from build123d import *

# Parameters (mm, degrees)
SKETCH1_R           = 15
BOSS_EXTRUDE1_DEPTH = 15


with BuildPart() as part:
    # Sketch1 → Boss-Extrude1 (new, symmetric)
    with BuildSketch(Plane.XY):
        with BuildLine():
            Line((0, 0), (0, 106))
            ThreePointArc((0, 106), (1.171572875, 108.828427125), (4, 110))
            Line((4, 110), (56, 110))
            ThreePointArc((56, 110), (58.828427125, 108.828427125), (60, 106))
            Line((60, 106), (60, 83.851648071))
            ThreePointArc((60, 83.851648071), (61.068687565, 81.129992802), (63.703703704, 79.862637103))
            ThreePointArc((63.703703704, 79.862637103), (95.355339059, 65.355339059), (109.862637103, 33.703703704))
            ThreePointArc((109.862637103, 33.703703704), (111.129992802, 31.068687565), (113.851648071, 30))
            Line((113.851648071, 30), (151, 30))
            ThreePointArc((151, 30), (153.828427125, 28.828427125), (155, 26))
            Line((155, 26), (155, 0))
            Line((155, 0), (0, 0))
        make_face()
        with Locations((30, 80)):
            Circle(SKETCH1_R, mode=Mode.SUBTRACT)
        with BuildLine():
            Line((85.690465157, 30), (24, 30))
            ThreePointArc((24, 30), (21.171572875, 31.171572875), (20, 34))
            Line((20, 34), (20, 56))
            ThreePointArc((20, 56), (21.171572875, 58.828427125), (24, 60))
            Line((24, 60), (60, 60))
            ThreePointArc((60, 60), (79.513309068, 52.786635759), (89.642844412, 34.615384615))
            ThreePointArc((89.642844412, 34.615384615), (88.728683259, 31.398225458), (85.690465157, 30))
        make_face(mode=Mode.SUBTRACT)
    extrude(amount=BOSS_EXTRUDE1_DEPTH, both=True)


solid = part.part
Check sheet for the modelled part. Datum: model origin and axes. Units: mm. A direction names the side the tool comes from. Coordinates: 2 decimals unless noted, no trailing zeros. Loops run counter-clockwise (first coordinate to the right, second up) from the corner with the lowest first, then second, coordinate; pieces in that order, holes last. Notation, with made-up numbers: (34, 55.5) -> (60, 55.5) arc R25 ccw to (60, 81.5) -> close; hole circle Ø7 at (83.25, 75.25). An arc over 180 degrees is marked (long way). Answer in a Markdown table with one row per item.
1. Sectioned sample at D-D, the plane x = 132. Record the boundary of the cut face in (y, z), then the cut area to 3 significant figures.
Check values:
| item | result |
|---|---|
| outline | (0, -15) -> (30, -15) -> (30, 15) -> (0, 15) -> close |
| area | 900 mm2 |
2. Sectioned sample at C-C, the plane y = 47.5. Record the boundary of the cut face in (x, z), then the cut area to 3 significant figures.
Check values:
| item | result |
|---|---|
| outline | (0, -15) -> (20, -15) -> (20, 15) -> (0, 15) -> close; (84.37, -15) -> (106.84, -15) -> (106.84, 15) -> (84.37, 15) -> close |
| area | 1,270 mm2 |
3. Sectioned sample at B-B, the plane z = -6. Record the boundary of the cut face in (x, y), then the cut area to 3 significant figures.
Check values:
| item | result |
|---|---|
| outline | (0, 0) -> (155, 0) -> (155, 26) arc R4 ccw to (151, 30) -> (113.85, 30) arc R4 cw to (109.86, 33.7) arc R50 ccw to (63.7, 79.86) arc R4 cw to (60, 83.85) -> (60, 106) arc R4 ccw to (56, 110) -> (4, 110) arc R4 ccw to (0, 106) -> close; hole circle Ø30 at (30, 80); hole (20, 34) arc R4 ccw to (24, 30) -> (85.69, 30) arc R4 ccw to (89.64, 34.62) arc R30 ccw to (60, 60) -> (24, 60) arc R4 ccw to (20, 56) -> close |
| area | 8,810 mm2 |
4. Material ranges on line 1 along Y through (x, z) = (30, 3.75); line 2 along X through (y, z) = (73, 7); line 3 along X through (y, z) = (100.5, -6.75), recorded low to high. Write a range as [from, to].
Check values:
| item | result |
|---|---|
| line 1 | y = [0, 30], [60, 65], [95, 110] |
| line 2 | x = [0, 16.73], [43.27, 85.51] |
| line 3 | x = [0, 60] |
5. Access from +Z, -Z, +X, -X, +Y, -Y to the whole of each face (thin tool, end or side, straight path). Record for faces 1 (the face through (55, 30, 0)), 2 (the face through (30, 110, 0)).
Check values:
| item | result |
|---|---|
| face 1 | +Z, -Z |
| face 2 | +Z, -Z, +X, -X, +Y |
6. Go/stop test with flat-tipped pins: pin 1 (10 mm diameter, centred on x = 47.5, z = -6, fed in from -Y); pin 2 (11 mm diameter, centred on y = 49, z = -1.5, fed in from +X); pin 3 (6.5 mm diameter, centred on y = 92.5, z = -5, fed in from +X). Record where each tip stops, or that it passes through.
Check values:
| item | result |
|---|---|
| pin 1 | stops at y = 0 |
| pin 2 | stops at x = 108.14 |
| pin 3 | stops at x = 60 |
7. Release check for a two-part mould opening along X. For faces 3 (the face through (60, 95, 0)), 4 (the face through (61, 19, -15)), 5 (the face through (79.286, 52.979, 0.21)), 6 (the face through (0, 52, 0)) record: released by +X, released by -X, zero draft, split by the parting line, or undercut.
Check values:
| item | result |
|---|---|
| face 3 | released by +X |
| face 4 | zero draft |
| face 5 | undercut |
| face 6 | released by -X |
8. Sectioned sample at A-A, the plane x = 30. Record the boundary of the cut face in (y, z).
Check values:
| item | result |
|---|---|
| outline | (0, -15) -> (30, -15) -> (30, 15) -> (0, 15) -> close; (60, -15) -> (65, -15) -> (65, 15) -> (60, 15) -> close; (95, -15) -> (110, -15) -> (110, 15) -> (95, 15) -> close |
